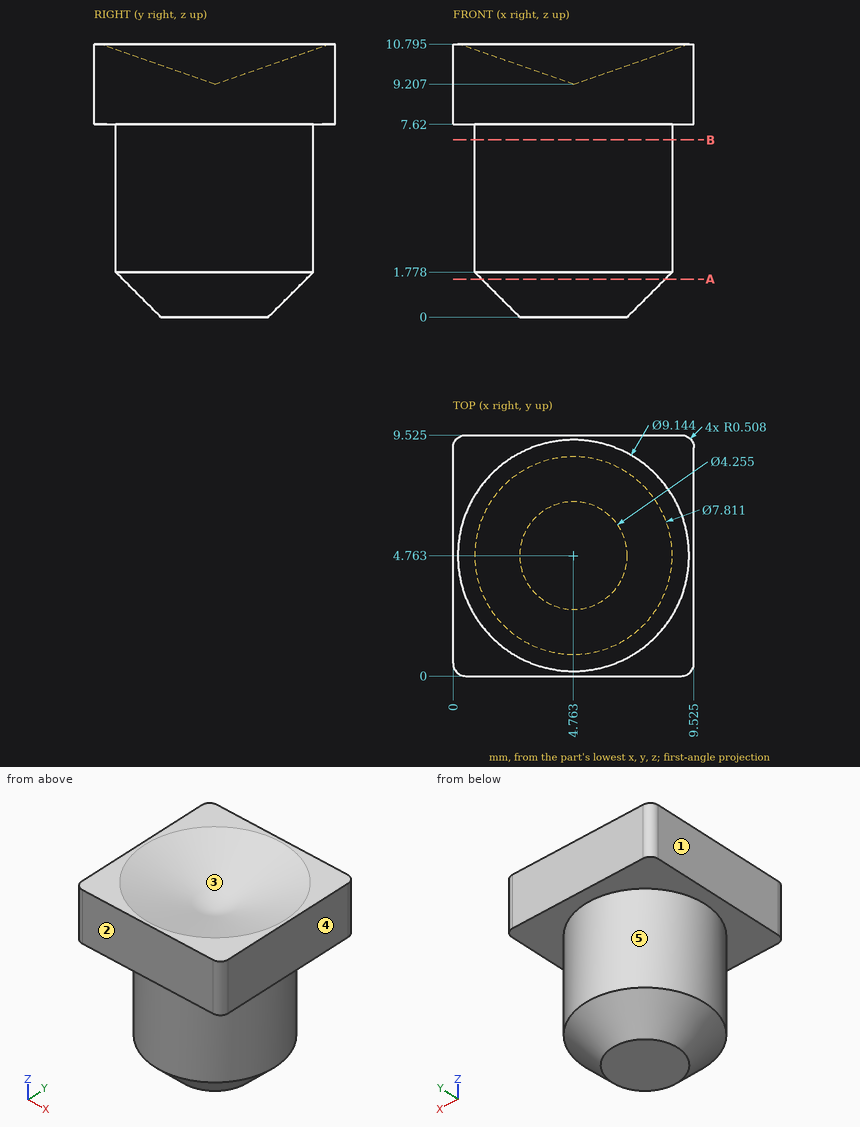
Job drawing, mm, ordinate dimensions from the low corner. One solid piece. A direction names the side the tool comes from. Round coordinates to 2 decimals unless told otherwise and drop trailing zeros. Loops run counter-clockwise (first coordinate to the right, second up) from the corner with the lowest first, then second, coordinate; pieces in that order, holes last.
(1) Drop flat-ended pins along their axis: pin 1 (3 mm diameter, centred on x = 3, z = 3.5, fed in from +Y); pin 2 (2 mm diameter, centred on x = 8.5, z = 5.5, fed in from +Y). Give the stop position or say it passes through.
(2) Which spindle directions (+Z, -Z, +X, -X, +Y, -Y) get a long thin tool onto all of the face, cutting with end or side? Do the marked faces 4 and 5. Say none if no direction does.
(3) Wall check: line 1 along Z through (x, y) = (1, 1.5) (1 decimal); line 2 along Y through (x, z) = (4.25, 4.25) (1 decimal); line 3 along Y through (x, z) = (1.25, 3.5) (1 decimal). Give the ranges that are in metal, low to high.
(4) Cut at A-A (z = 1.5). Give the cut face in (x, y) (1 decimal).
(5) Cut at B-B (z = 7). Give the cut face in (x, y) (1 decimal), plus the area to 3 significant figures.
(6) Two-plate mould, pull along Y, no slides. Class the marked faces 1, 2 and 3: +Y half, -Y half, draft (parallel to the pull), parting line (faces both ways), or undercut.
Findings below:
1. pin 1: stops at y = 8.66
1. pin 2: stops at y = 7.55
2. face 4: +Z, -Z, +X, +Y, -Y
2. face 5: -Z
3. line 1: z = 7.6 to 10.8
3. line 2: y = 0.9 to 8.6
3. line 3: y = 3.1 to 6.5
4. outline: circle Ø7.3 at (4.8, 4.8)
5. outline: circle Ø7.8 at (4.8, 4.8)
5. area: 47.9 mm2
6. face 1: draft
6. face 2: -Y half
6. face 3: undercut
